The listing builds one solid part. Answer for the finished solid, in the listing's coordinates (mm). Face numbers are marked on the shaded views. A direction names the side the tool comes from. Round coordinates to 2 decimals unless told otherwise and drop trailing zeros. Write each loop counter-clockwise with the first axis right and the second up, starting at its lowest first coordinate (ties: lowest second). Pieces come first, ordered by that corner, then holes.
from build123d import *

# Parameters (mm, degrees)
SKIZZE1_W                       = 50
SKIZZE1_H                       = 52
SKIZZE1_R                       = 8.8
SKIZZE1_R_2                     = 2.25
AUFSATZ_LINEAR_AUSTRAGEN1_DEPTH = 3
SKIZZE2_W                       = 50
SKIZZE2_H                       = 2.999801306
AUFSATZ_LINEAR_AUSTRAGEN2_DEPTH = 52
SCHNITT_LINEAR_AUSTRAGEN1_DEPTH = 78.788299069


with BuildPart() as part:
    # Skizze1 → Aufsatz-Linear austragen1 (new body)
    with BuildSketch(Plane.XY):
        Rectangle(SKIZZE1_W, SKIZZE1_H)
        with Locations((0, 2)):
            Circle(SKIZZE1_R, mode=Mode.SUBTRACT)
        with Locations((-14.5, 2)):
            Circle(SKIZZE1_R_2, mode=Mode.SUBTRACT)
        with Locations((14.5, 2)):
            Circle(SKIZZE1_R_2, mode=Mode.SUBTRACT)
    extrude(amount=AUFSATZ_LINEAR_AUSTRAGEN1_DEPTH)

    # Skizze2 → Aufsatz-Linear austragen2 (add)
    with BuildSketch(Plane.XY.offset(3)):
        with Locations((0, -24.500099347)):
            Rectangle(SKIZZE2_W, SKIZZE2_H)
    extrude(amount=AUFSATZ_LINEAR_AUSTRAGEN2_DEPTH)

    # Skizze3 → Schnitt-Linear austragen1 (cut, through all)
    with BuildSketch(Plane(origin=(0, -23.000198694, 0), x_dir=(1, 0, 0), z_dir=(0, 1, 0))):
        with BuildLine():
            Line((-14.25, -36.75), (-8.75, -36.75))
            ThreePointArc((-8.75, -36.75), (-6.5, -39), (-8.75, -41.25))
            Line((-8.75, -41.25), (-14.25, -41.25))
            ThreePointArc((-14.25, -41.25), (-16.5, -39), (-14.25, -36.75))
        make_face()
        with BuildLine():
            Line((8.75, -36.75), (14.25, -36.75))
            ThreePointArc((14.25, -36.75), (16.5, -39), (14.25, -41.25))
            Line((14.25, -41.25), (8.75, -41.25))
            ThreePointArc((8.75, -41.25), (6.5, -39), (8.75, -36.75))
        make_face()
        with BuildLine():
            Line((-14.25, -8.75), (-8.75, -8.75))
            ThreePointArc((-8.75, -8.75), (-6.5, -11), (-8.75, -13.25))
            Line((-8.75, -13.25), (-14.25, -13.25))
            ThreePointArc((-14.25, -13.25), (-16.5, -11), (-14.25, -8.75))
        make_face()
        with BuildLine():
            Line((8.75, -8.75), (14.25, -8.75))
            ThreePointArc((14.25, -8.75), (16.5, -11), (14.25, -13.25))
            Line((14.25, -13.25), (8.75, -13.25))
            ThreePointArc((8.75, -13.25), (6.5, -11), (8.75, -8.75))
        make_face()
    extrude(amount=-SCHNITT_LINEAR_AUSTRAGEN1_DEPTH, mode=Mode.SUBTRACT)


solid = part.part
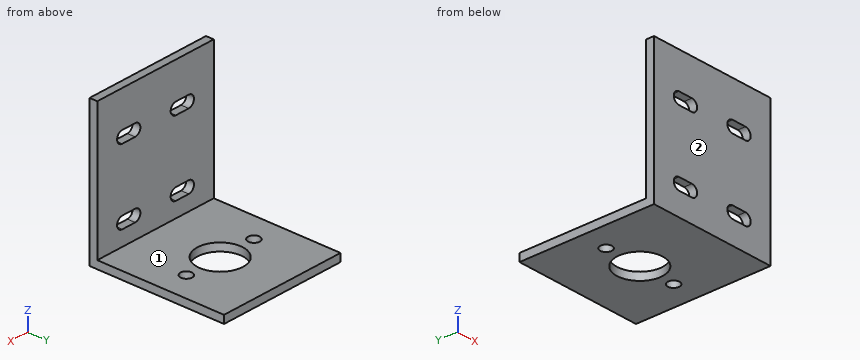
1. Section A-A on z = 11 is taken. Determine the outline of the cut face in (x, y).
Geometry says:
outline: (-25, -26) - (-16.5, -26) - (-16.5, -23) - (-25, -23) - close; (-6.5, -26) - (6.5, -26) - (6.5, -23) - (-6.5, -23) - close; (16.5, -26) - (25, -26) - (25, -23) - (16.5, -23) - close
2. A tool of negligible diameter and unlimited length cuts with its end or side. For the marked faces 1 and 2, from which of +Z, -Z, +X, -X, +Y, -Y can it reach the whole face along a straight path? Write none if from no direction.
Geometry says:
face 1: +Z, +X, -X, +Y
face 2: +Z, -Z, +X, -X, -Y
3. Section B-B on y = 2 is taken. Determine the outline of the cut face in (x, z).
Geometry says:
outline: (-25, 0) - (-16.75, 0) - (-16.75, 3) - (-25, 3) - close; (-12.25, 0) - (-8.8, 0) - (-8.8, 3) - (-12.25, 3) - close; (8.8, 0) - (12.25, 0) - (12.25, 3) - (8.8, 3) - close; (16.75, 0) - (25, 0) - (25, 3) - (16.75, 3) - close
4. Section C-C on x = 0 is taken. Determine the outline of the cut face in (y, z), plus the area to 3 significant figures.
Geometry says:
outline: (-26, 0) - (-6.8, 0) - (-6.8, 3) - (-23, 3) - (-23, 55) - (-26, 55) - close; (10.8, 0) - (26, 0) - (26, 3) - (10.8, 3) - close
area: 259 mm2
5. Section D-D on x = 13.5 is taken. Determine the outline of the cut face in (y, z).
Geometry says:
outline: (-26, 0) - (-0.02, 0) - (-0.02, 3) - (-23, 3) - (-23, 8.75) - (-26, 8.75) - close; (-26, 13.25) - (-23, 13.25) - (-23, 36.75) - (-26, 36.75) - close; (-26, 41.25) - (-23, 41.25) - (-23, 55) - (-26, 55) - close; (4.02, 0) - (26, 0) - (26, 3) - (4.02, 3) - close
6. Given pin 1 (12 mm diameter, centred on x = -8, z = 28.5, fed in from +Y); pin 2 (23 mm diameter, centred on x = 0, y = 2, fed in from +Z), each flat-ended and moving along its own axis, determine where each tip first touches the part or whether it passes through.
Geometry says:
pin 1: stops at y = -23
pin 2: stops at z = 3
7. Straight lines are drawn through the part: line 1 along Y through (x, z) = (-14.5, 0.85); line 2 along Z through (x, y) = (12, 9); line 3 along Y through (x, z) = (-6, 20). For each, find the intervals that lie inside material, in ascending order.
Geometry says:
line 1: y = -26 to -0.25, 4.25 to 26
line 2: z = 0 to 3
line 3: y = -26 to -23
